Source: CAD feature listing. Evaluate the final solid. Frame: model axes, mm. Coordinates: 2 decimals unless noted, no trailing zeros. Write each loop counter-clockwise with the first axis right and the second up, starting at its lowest first coordinate (ties: lowest second). Pieces come first, ordered by that corner, then holes. Notation, with made-up numbers: (-13.5, -2) -> (-4.5, -2) arc R15 cw to (-4.5, 26) -> close; hole circle Ø7 at (-31.5, 10). An arc over 180 degrees is marked (long way). One line per item, written item: value. Start each with the question number.
1. Section query A-A, the plane y = -156. Output: boundary loops of the cut face in (x, z), and give its area (3 significant figures).
2. Section query D-D, the plane z = 1.65. State how many separate pieces and enclosed holes the cut face has, and give its area (3 significant figures).
3. First-contact query: P1, Ø2, axis at y = -48, z = 2, coming from the -X side; P2, Ø3, axis at y = -151.5, z = 0.5, coming from the +X side. Flat tips, straight axial feed; report the tip coordinate or a pass-through.
4. Section query C-C, the plane y = -118.95. Output: boundary loops of the cut face in (x, z), and give its area (3 significant figures).
5. Section query B-B, the plane x = 25. Output: boundary loops of the cut face in (y, z), and give its area (3 significant figures).
6. Line query: line 1 (X direction, y = -181, z = 2.95); line 2 (Y direction, x = 60, z = 3.5); line 3 (X direction, y = -131, z = 3.3). Output: solid intervals per line, ascending.
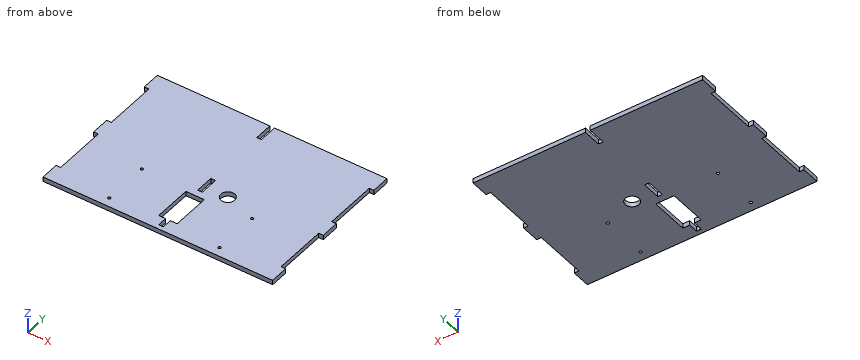
from build123d import *

# Parameters (mm, degrees)
BOSS_EXTRU_1_OUTLINE_W  = 5
BOSS_EXTRU_1_OUTLINE_H  = 20
BOSS_EXTRU_1_DEPTH      = 5
ESQUISSE2_R             = 1.5
ENL_V_MAT_EXTRU_1_DEPTH = 229.322140845
ESQUISSE3_R             = 7.5
ENL_V_MAT_EXTRU_2_DEPTH = 229.322140845


# Read off the part's stored shape, not the designer's step: Boss.-Extru.1
with BuildPart() as part:
    # Boss.-Extru.1 outline → Boss.-Extru.1 (new body)
    with BuildSketch(Plane.XY):
        Polygon((125, -16), (2.5, -16), (2.5, -36), (-2.5, -36), (-2.5, -16), (-125, -16), (-125, -36), (-120, -36), (-120, -93.5), (-125, -93.5), (-125, -113.5), (-120, -113.5), (-120, -171), (-125, -171), (-125, -191), (125, -191), (125, -171), (120, -171), (120, -113.5), (125, -113.5), (125, -93.5), (120, -93.5), (120, -36), (125, -36), align=None)
        Polygon((10, -133.95), (10, -175.45), (2.5, -175.45), (2.5, -186), (-2.5, -186), (-2.5, -175.45), (-10, -175.45), (-10, -133.95), align=None, mode=Mode.SUBTRACT)
        with Locations((0, -116.4)):
            Rectangle(BOSS_EXTRU_1_OUTLINE_W, BOSS_EXTRU_1_OUTLINE_H, mode=Mode.SUBTRACT)
    extrude(amount=BOSS_EXTRU_1_DEPTH)

    # Esquisse2 → Enlèv. mat.-Extru.1 (cut, through all)
    with BuildSketch(Plane.XY.offset(5)):
        with Locations((60, -131)):
            Circle(ESQUISSE2_R)
        with Locations((60, -181)):
            Circle(ESQUISSE2_R)
        with Locations(Location((-60, -131, 0), (0, 0, 180))):
            Circle(ESQUISSE2_R)
        with Locations(Location((-60, -181, 0), (0, 0, 180))):
            Circle(ESQUISSE2_R)
    extrude(amount=-ENL_V_MAT_EXTRU_1_DEPTH, mode=Mode.SUBTRACT)

    # Esquisse3 → Enlèv. mat.-Extru.2 (cut, through all)
    with BuildSketch(Plane.XY.offset(5)):
        with Locations((25, -118.95)):
            Circle(ESQUISSE3_R)
    extrude(amount=-ENL_V_MAT_EXTRU_2_DEPTH, mode=Mode.SUBTRACT)


solid = part.part
Computed values:
1. outline: (-120, 0) -> (-10, 0) -> (-10, 5) -> (-120, 5) -> close; (10, 0) -> (120, 0) -> (120, 5) -> (10, 5) -> close
1. area: 1,100 mm²
2. separate pieces: 1
2. enclosed holes: 7
2. area: 41,300 mm²
3. P1: stops at x = -120
3. P2: stops at x = 120
4. outline: (-120, 0) -> (-2.5, 0) -> (-2.5, 5) -> (-120, 5) -> close; (2.5, 0) -> (17.5, 0) -> (17.5, 5) -> (2.5, 5) -> close; (32.5, 0) -> (120, 0) -> (120, 5) -> (32.5, 5) -> close
4. area: 1,100 mm²
5. outline: (-191, 0) -> (-126.45, 0) -> (-126.45, 5) -> (-191, 5) -> close; (-111.45, 0) -> (-16, 0) -> (-16, 5) -> (-111.45, 5) -> close
5. area: 800 mm²
6. line 1: x = -125 to -61.5, -58.5 to -2.5, 2.5 to 58.5, 61.5 to 125
6. line 2: y = -191 to -182.5, -179.5 to -132.5, -129.5 to -16
6. line 3: x = -120 to -61.5, -58.5 to 58.5, 61.5 to 120
